Work out the finished part from the listing and answer in its coordinate system (mm). A direction names the side the tool comes from. Coordinates: 2 decimals unless noted, no trailing zeros. Order: outer loops, then holes, each group sorted by start corner. A loop starts at its lowest first (then second) coordinate and runs counter-clockwise, first axis right, second up. Notation, with made-up numbers: M 52.5,70.25 L 102.5,70.25 A23 cw 102.5,89.25 Z; hole C -25,-30.75 d11. An arc over 180 degrees is marked long. Use a Markdown table: item, result.
from build123d import *

# Parameters (mm, degrees)
SKETCH_1_R          = 24
SKETCH_1_R_2        = 20
EXTRUDE_1_DEPTH     = 24
SKETCH_2_R          = 29
SKETCH_2_R_2        = 24
EXTRUDE_2_DEPTH     = 5
SKETCH_3_W          = 29
SKETCH_3_H          = 58
CUT_EXTRUDE_1_DEPTH = 49
CHAMFER_1_SIZE      = 1


with BuildPart() as part:
    # Эскиз1 → Бобышка-Вытянуть1 (new body)
    with BuildSketch(Plane.XY):
        Circle(SKETCH_1_R)
        Circle(SKETCH_1_R_2, mode=Mode.SUBTRACT)
    extrude(amount=EXTRUDE_1_DEPTH)

    # Эскиз2 → Бобышка-Вытянуть2 (add)
    with BuildSketch(Plane.XY.offset(24)):
        Circle(SKETCH_2_R)
        Circle(SKETCH_2_R_2, mode=Mode.SUBTRACT)
    extrude(amount=-EXTRUDE_2_DEPTH)

    # Зеркальное отражение1: part across plane


with BuildPart() as part_1:
    add(part.part)
    add(part.part.mirror(Plane.XY))

    # Эскиз3 → Вырез-Вытянуть1 (cut, through all)
    with BuildSketch(Plane.XY.offset(24)):
        with Locations((14.5, 0)):
            Rectangle(SKETCH_3_W, SKETCH_3_H)
    extrude(amount=-CUT_EXTRUDE_1_DEPTH, mode=Mode.SUBTRACT)

    # Фаска1
    chamfer_1_edges = [part_1.edges().sort_by_distance(p)[0] for p in [
        (-29, 0, -24),
        (-29, 0, 24),
    ]]
    chamfer(chamfer_1_edges, length=CHAMFER_1_SIZE)


solid = part_1.part
1. For a pull along Z with two mould halves and no side action, classify faces 3 (the face through (-20.4, 0.4, -24)), 4 (the face through (-28.153, 0.619, 23.84)), 5 (the face through (-23.994, 0.528, 0.266)) as +Z half, -Z half, draft (parallel to the pull), parting line (faces both ways), or undercut.
Answers below:
| item | result |
|---|---|
| face 3 | -Z half |
| face 4 | +Z half |
| face 5 | undercut |
2. Find the intervals of material crossed by probe 1 along Z at (x, y) = (-9.75, 24.5); probe 2 along X at (y, z) = (0, -4); probe 3 along Y at (x, z) = (-15, 9.5) (3 decimals), in increasing order.
Answers below:
| item | result |
|---|---|
| probe 1 | -24 to -19, 19 to 24 |
| probe 2 | -24 to -20 |
| probe 3 | -18.735 to -13.229, 13.229 to 18.735 |
3. Flat-ended cylindrical pins translate along their axes: P1, Ø2, axis at x = -13, z = -4.5, coming from the +Y side; P2, Ø5, axis at x = -15, z = -19, coming from the -Y side; P3, Ø12, axis at y = 6.5, z = 9, coming from the +X side. Find the tip coordinate at first contact, or state that the pin passes through.
Answers below:
| item | result |
|---|---|
| P1 | y = 20.78 |
| P2 | y = -26.17 |
| P3 | x = -15.61 |
4. Section C-C on z = 9 is taken. Determine the outline of the cut face in (x, y).
Answers below:
| item | result |
|---|---|
| outline | M 0,-24 L 0,-20 A20 cw 0,20 L 0,24 A24 ccw Z |
5. Section B-B on z = 21.5 is taken. Determine the outline of the cut face in (x, y), then the cut area to 3 significant figures.
Answers below:
| item | result |
|---|---|
| outline | M 0,-29 L 0,-20 A20 cw 0,20 L 0,29 A29 ccw Z |
| area | 693 mm² |
6. For faces 1 (the face through (-24.2, 0.1, -19)), 2 (the face through (-28.993, 0.638, 21.028)), determine the directions among +Z, -Z, +X, -X, +Y, -Y from which every point of the face is accessible in a straight line to the end or side of a thin tool.
Answers below:
| item | result |
|---|---|
| face 1 | -X |
| face 2 | +Z, -Z, -X |
7. Section A-A on y = 0 is taken. Determine the outline of the cut face in (x, z), then the cut area to 3 significant figures.
Answers below:
| item | result |
|---|---|
| outline | M -29,-23 L -28,-24 L -20,-24 L -20,24 L -28,24 L -29,23 L -29,19 L -24,19 L -24,-19 L -29,-19 Z |
| area | 241 mm² |
